Autodesk Inventor part; units mm, degrees
ref_plane "YZ Plane" through (0, 0, 0) normal (1, 0, 0) x (0, 1, 0)
ref_plane "XZ Plane" through (0, 0, 0) normal (0, 1, 0) x (-1, 0, 0)
ref_plane "XY Plane" through (0, 0, 0) normal (0, 0, 1) x (1, 0, 0)
sketch "Sketch2" plane through (0, 0, 0) normal (0, 0, 1) x (1, 0, 0)
  line L0 (0, 0) -> (0, 4.9506) construction
  line L1 (-8.5, -5) -> (-6, -5)
  line L2 (-6, -5) -> (-6, 5)
  line L3 (-6, 5) -> (-8.5, 5)
  line L4 (-8.5, 5) -> (-8.5, -5)
  line L5 (-8.5, -5) -> (-6, 5) construction
  line L6 (-6, -5) -> (-8.5, 5) construction
  line L7 (-16, -5) -> (-13.5, -5)
  line L8 (-13.5, -5) -> (-13.5, 5)
  line L9 (-13.5, 5) -> (-16, 5)
  line L10 (-16, 5) -> (-16, -5)
  line L11 (-16, -5) -> (-13.5, 5) construction
  line L12 (-13.5, -5) -> (-16, 5) construction
  line L13 (-13.5, -4.5) -> (-8.5, -4.5)
  line L14 (-8.5, -4.5) -> (-8.5, 4.5)
  line L15 (-8.5, 4.5) -> (-13.5, 4.5)
  line L16 (-13.5, 4.5) -> (-13.5, -4.5)
  line L17 (-13.5, -4.5) -> (-8.5, 4.5) construction
  line L18 (-8.5, -4.5) -> (-13.5, 4.5) construction
  point P0 (-7.25, 0)
  point P1 (-14.75, 0)
  point P2 (-11, 0)
  point P3 (-14.75, 0)
  point P4 (-7.25, 0)
  dimension "d11" = 12
  dimension "d12" = 32
  dimension "d13" = 2.5
  dimension "d14" = 2.5
  dimension "d15" = 10
  dimension "d16" = 9
revolve "Revolution1" add sketch "Sketch2" angle 360 about axis through (0, 0, 0) along (0, 1, 0)
properties part number "P03 - Bearing 62012" material "SAE 1020"
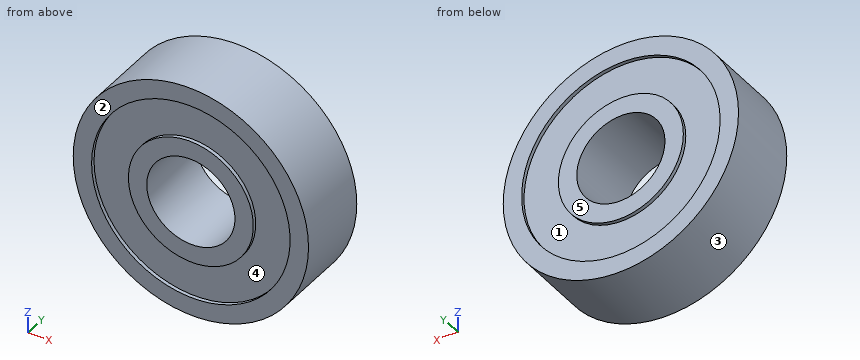
Model file for the job. Use its own axes, mm. Face numbers are marked on the shaded views. A direction names the side the tool comes from. Round coordinates to 2 decimals unless told otherwise and drop trailing zeros. Write each loop counter-clockwise with the first axis right and the second up, starting at its lowest first coordinate (ties: lowest second). Pieces come first, ordered by that corner, then holes. Notation, with made-up numbers: (47, 0.5) - (92, 0.5) arc R7 cw to (92, 12.5) - close; hole circle Ø1 at (27, 24.25). An arc over 180 degrees is marked (long way). One line per item, written item: value.
(1) Cut at B-B, the plane z = 0. Give the cut face in (x, y).
Values follow:
outline: (-16, -5) - (-13.5, -5) - (-13.5, -4.5) - (-8.5, -4.5) - (-8.5, -5) - (-6, -5) - (-6, 5) - (-8.5, 5) - (-8.5, 4.5) - (-13.5, 4.5) - (-13.5, 5) - (-16, 5) - close; (6, -5) - (8.5, -5) - (8.5, -4.5) - (13.5, -4.5) - (13.5, -5) - (16, -5) - (16, 5) - (13.5, 5) - (13.5, 4.5) - (8.5, 4.5) - (8.5, 5) - (6, 5) - close
(2) Cut at A-A, the plane x = -1. Give the cut face in (y, z).
Values follow:
outline: (-5, -15.97) - (5, -15.97) - (5, -13.46) - (4.5, -13.46) - (4.5, -8.44) - (5, -8.44) - (5, -5.92) - (-5, -5.92) - (-5, -8.44) - (-4.5, -8.44) - (-4.5, -13.46) - (-5, -13.46) - close; (-5, 5.92) - (5, 5.92) - (5, 8.44) - (4.5, 8.44) - (4.5, 13.46) - (5, 13.46) - (5, 15.97) - (-5, 15.97) - (-5, 13.46) - (-4.5, 13.46) - (-4.5, 8.44) - (-5, 8.44) - close
(3) Cut at C-C, the plane y = 3.5. Give the cut face in (x, z).
Values follow:
outline: circle Ø32 at (0, 0); hole circle Ø12 at (0, 0)
(4) 3-axis set-ups, long thin cutter, end or side, ignore diameter. For the marked faces 4 and 5: which of +Z, -Z, +X, -X, +Y, -Y reach the whole face in a straight line?
Values follow:
face 4: -Y
face 5: +Z, -Z, +X, -X, +Y
(5) Cut at D-D, the plane z = 9. Give the cut face in (x, y), plus the area to 3 significant figures.
Values follow:
outline: (-13.23, -5) - (-10.06, -5) - (-10.06, -4.5) - (10.06, -4.5) - (10.06, -5) - (13.23, -5) - (13.23, 5) - (10.06, 5) - (10.06, 4.5) - (-10.06, 4.5) - (-10.06, 5) - (-13.23, 5) - close
area: 244 mm²
(6) Wall check: probe 1 along Z at (x, y) = (0, 4.65); probe 2 along Z at (x, y) = (0, -2); probe 3 along X at (y, z) = (0.5, -5.5). Give the ranges that are in metal, low to high.
Values follow:
probe 1: z = -16 to -13.5, -8.5 to -6, 6 to 8.5, 13.5 to 16
probe 2: z = -16 to -6, 6 to 16
probe 3: x = -15.02 to -2.4, 2.4 to 15.02
(7) Drop flat-ended pins along their axis: P1, Ø6, axis at x = 12, y = -3, coming from the -Z side; P2, Ø4, axis at y = -1, z = 11, coming from the +X side; P3, Ø4, axis at y = -3.5, z = -10.5, coming from the -X side. Give the stop position or say it passes through.
Values follow:
P1: stops at z = -13.23
P2: stops at x = 13.23
P3: stops at x = -13.56
(8) Two-plate mould, pull along X, no slides. Class the marked faces 1, 2 and 3: pulls with the +X half, pulls with the -X half, needs draft (parallel to the pull), parting line crosses it, or undercut.
Values follow:
face 1: undercut
face 2: needs draft
face 3: parting line crosses it
